```python
from build123d import *

# Parameters (mm, degrees)
F0_W      = 127
F0_H      = 50.8
F1_DEPTH  = 19.05
F2_W      = 88.9
F2_H      = 17.78
F3_DEPTH  = 165.1
F4_W      = 13.97
F4_H      = 154.94
F5_DEPTH  = 100.584
F6_W      = 88.9
F6_H      = 1.27
F7_DEPTH  = 24.13
F8_W      = 1.27
F8_H      = 19.05
F9_DEPTH  = 165.1
F10_DEPTH = 1.27


with BuildPart() as f1:
    # F0 (on Top) → F1 (new body)
    with BuildSketch(Plane.XY):
        with Locations((63.5, 25.4)):
            Rectangle(F0_W, F0_H)
    extrude(amount=F1_DEPTH)

    # F2 (on face) → F3 (join)
    with BuildSketch(Plane.XY.offset(19.05)):
        with Locations((63.5, 26.67)):
            Rectangle(F2_W, F2_H)
    extrude(amount=F3_DEPTH)

    # F4 (on face) → F5 (cut)
    with BuildSketch(Plane.YZ.offset(107.95)):
        with Locations((24.765, 101.6)):
            Rectangle(F4_W, F4_H)
    extrude(amount=-F5_DEPTH, mode=Mode.SUBTRACT)

    # F6 (on face) → F7 (join)
    with BuildSketch(Plane.XY.offset(19.05)):
        with Locations((63.5, 17.145)):
            Rectangle(F6_W, F6_H)
    extrude(amount=F7_DEPTH)

    # F8 (on face) → F9 (join)
    with BuildSketch(Plane.XY.offset(19.05)):
        with Locations((108.585, 26.035)):
            Rectangle(F8_W, F8_H)
    extrude(amount=F9_DEPTH)

    # F10 (add): a face of the model
    f10_faces = [f1.faces().sort_by_distance(p)[0] for p in [
        (63.5, 17.78, 181.61),
    ]]
    extrude(f10_faces, amount=F10_DEPTH)


solid = f1.part
```
Work out the finished part from the listing and answer in its coordinate system (mm). A direction names the side the tool comes from. Coordinates: 2 decimals unless noted, no trailing zeros. Loops run counter-clockwise (first coordinate to the right, second up) from the corner with the lowest first, then second, coordinate; pieces in that order, holes last. Notation, with made-up numbers: (54.5, 72) -> (73.5, 72) arc R24 cw to (73.5, 88) -> close; hole circle Ø4 at (26.25, -17). An arc over 180 degrees is marked (long way). Answer as CSV lines item,"result".
Q1. The part is cut by section A-A on z = 30.5. Write down the section's boundary in (x, y), and give its area (3 significant figures).
Findings:
outline,"(19.05, 16.51) -> (109.22, 16.51) -> (109.22, 35.56) -> (19.05, 35.56) -> (19.05, 31.75) -> (107.95, 31.75) -> (107.95, 17.78) -> (19.05, 17.78) -> close"
area,"476 mm²"
Q2. For a pull along Z with two mould halves and no side action, classify faces 1 (the face through (64, 26, 184.15)), 2 (the face through (64, 25, 24.13)), 3 (the face through (64, 35.56, 100)) as +Z half, -Z half, draft (parallel to the pull), parting line (faces both ways), or undercut.
Findings:
face 1,"+Z half"
face 2,"undercut"
face 3,"draft"
Q3. The part is cut by section B-B on y = 21. Write down the section's boundary in (x, z), and give its area (3 significant figures).
Findings:
outline,"(0, 0) -> (127, 0) -> (127, 19.05) -> (109.22, 19.05) -> (109.22, 184.15) -> (19.05, 184.15) -> (19.05, 179.07) -> (107.95, 179.07) -> (107.95, 24.13) -> (19.05, 24.13) -> (19.05, 19.05) -> (0, 19.05) -> close"
area,"3,530 mm²"
Q4. The part is cut by section C-C on x = 103. Write down the section's boundary in (y, z), and give its area (3 significant figures).
Findings:
outline,"(0, 0) -> (50.8, 0) -> (50.8, 19.05) -> (35.56, 19.05) -> (35.56, 184.15) -> (16.51, 184.15) -> (16.51, 179.07) -> (31.75, 179.07) -> (31.75, 24.13) -> (17.78, 24.13) -> (17.78, 43.18) -> (16.51, 43.18) -> (16.51, 19.05) -> (0, 19.05) -> close"
area,"1,780 mm²"
Q5. The part is cut by section D-D on z = 63. Write down the section's boundary in (x, y).
Findings:
outline,"(19.05, 31.75) -> (107.95, 31.75) -> (107.95, 16.51) -> (109.22, 16.51) -> (109.22, 35.56) -> (19.05, 35.56) -> close"
Q6. Find the intervals of material crossed by probe 1 along Z at (x, y) = (40, 26); probe 2 along Y at (x, z) = (82, 175); probe 3 along X at (y, z) = (32, 111), in increasing order.
Findings:
probe 1,"z = 0 to 24.13, 179.07 to 184.15"
probe 2,"y = 31.75 to 35.56"
probe 3,"x = 19.05 to 109.22"
Q7. Each of these flat-tipped pins is pushed along its axis until it touches: pin 1 (12 mm diameter, centred on y = 32, z = 147.5, fed in from +X); pin 2 (9.5 mm diameter, centred on x = 74, z = 33.5, fed in from +Y); pin 3 (21 mm diameter, centred on y = 22, z = 140.5, fed in from -X); pin 4 (12 mm diameter, centred on y = 44, z = 156, fed in from +X). Where does it stop, or does it pass through?
Findings:
pin 1,"stops at x = 109.22"
pin 2,"stops at y = 35.56"
pin 3,"stops at x = 19.05"
pin 4,"passes through"
Q8. A tool of negligible diameter and unlimited length cuts with its end or side. For faces 4 (the face through (19.05, 32, 101)), 5 (the face through (64, 16.51, 40)), 6 (the face through (109.22, 26, 100)), from which of +Z, -Z, +X, -X, +Y, -Y can it reach the whole face along a straight path? Write none if from no direction.
Findings:
face 4,"+Z, -X, +Y, -Y"
face 5,"+Z, +X, -X, -Y"
face 6,"+Z, +X, +Y, -Y"
